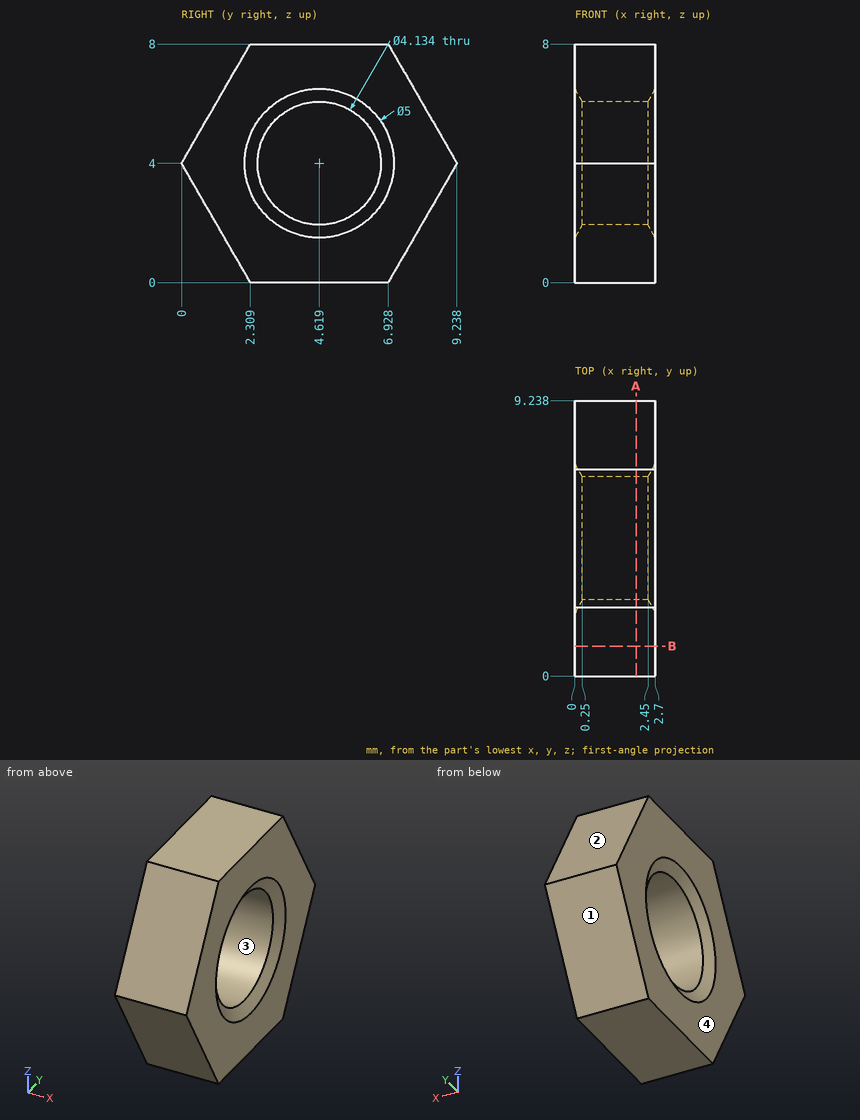
Geometry: see drawing. Coordinates: mm, zero at the bounding-box minimum. Round coordinates to 2 decimals unless told otherwise and drop trailing zeros. Loops run counter-clockwise (first coordinate to the right, second up) from the corner with the lowest first, then second, coordinate; pieces in that order, holes last. Notation, with made-up numbers: M -8.5,45 L 26.5,45 A29 ccw 26.5,84 Z; hole C 9.5,-3 d6. An arc over 180 degrees is marked long. Use a Markdown table: item, result. Add a question column.
1. Cut plane B-B, the plane y = 1. Output: boundary loops of the cut face in (x, z).
2. Ray query, line 1 along Y through (x, z) = (1.85, 4.25) (1 decimal); line 2 along Z through (x, y) = (1.4, 5.5); line 3 along Y through (x, z) = (1.2, 3.25) (1 decimal). Return the intervals inside material, ascending. Write a range as [from, to].
3. Pull-direction query (Z, two-part tool) for the marked faces 1, 2, 3 and 4; classes: +Z half, -Z half, draft (parallel to the pull), parting line (faces both ways), or undercut.
4. Cut plane A-A, the plane x = 2.05. Output: boundary loops of the cut face in (y, z).
Solution:
| question | item | result |
|---|---|---|
| 1 | outline | M 0,2.27 L 2.7,2.27 L 2.7,5.73 L 0,5.73 Z |
| 2 | line 1 | y = [0.1, 2.6], [6.7, 9.1] |
| 2 | line 2 | z = [0, 2.13], [5.87, 8] |
| 2 | line 3 | y = [0.4, 2.7], [6.5, 8.8] |
| 3 | face 1 | -Z half |
| 3 | face 2 | +Z half |
| 3 | face 3 | undercut |
| 3 | face 4 | draft |
| 4 | outline | M 0,4 L 2.31,0 L 6.93,0 L 9.24,4 L 6.93,8 L 2.31,8 Z; hole C 4.62,4 d4.13 |
